Could you check a few things on this model? Use its own coordinates, in mm. Face numbers are marked on the shaded views. A direction names the side the tool comes from. Coordinates: 2 decimals unless noted, no trailing zeros. Loops run counter-clockwise (first coordinate to the right, second up) from the corner with the lowest first, then second, coordinate; pieces in that order, holes last. Notation, with made-up numbers: M -10,30.25 L 30,30.25 A17 ccw 30,50.25 Z; hole C 63.25,4.25 d7. An arc over 180 degrees is marked long. Return JSON: item names as keys, results as strings. Group by question number.
from build123d import *

# Parameters (mm, degrees)
F0_W     = 65
F0_H     = 48.220679
F0_R     = 1.491954
F0_W_2   = 7.12351
F0_H_2   = 5.636183
F0_R_2   = 2.348409
F0_R_3   = 2.019025
F0_W_3   = 6.966946
F0_H_3   = 7.08437
F0_R_4   = 2.712275
F0_W_4   = 5.990132
F0_H_4   = 3.159632
F0_W_5   = 3.225457
F0_H_5   = 6.780042
F0_W_6   = 6.697657
F0_H_6   = 6.365542
F0_W_7   = 6.033428
F0_H_7   = 6.476249
F0_W_8   = 3.155096
F0_H_8   = 2.989037
F0_W_9   = 4.483557
F0_H_9   = 3.376505
F0_W_10  = 5.864762
F0_H_10  = 13.520941
F1_DEPTH = 1.5
F2_DEPTH = 2
F3_DEPTH = 4
F4_DEPTH = 7
F5_W     = 2.606562
F5_H     = 14.894642
F5_W_2   = 2.66153
F5_H_2   = 7.59319
F5_W_3   = 15.029821
F5_H_3   = 2.42669
F5_W_4   = 15.577784
F5_H_4   = 2.504971
F6_DEPTH = 7


with BuildPart() as f1:
    # F0 (on Top) → F1 (new body)
    with BuildSketch(Plane.XY):
        with Locations((15.373986, 7.248863)):
            Rectangle(F0_W, F0_H)
        with Locations((-13.490251, -13.718908)):
            Circle(F0_R, mode=Mode.SUBTRACT)
        with Locations((-6.637482, -5.545355)):
            Rectangle(F0_W_2, F0_H_2, mode=Mode.SUBTRACT)
        with Locations((16.112888, -10.907532)):
            Circle(F0_R_2, mode=Mode.SUBTRACT)
        with Locations((45.080185, -12.724719)):
            Circle(F0_R_3, mode=Mode.SUBTRACT)
        with Locations((33.124202, 5.70149)):
            Rectangle(F0_W_3, F0_H_3, mode=Mode.SUBTRACT)
        with Locations((-12.451392, 11.686808)):
            Circle(F0_R_4, mode=Mode.SUBTRACT)
        with Locations((-5.081796, 11.177822)):
            Rectangle(F0_W_4, F0_H_4, mode=Mode.SUBTRACT)
        with Locations((5.516132, 11.934817)):
            Rectangle(F0_W_5, F0_H_5, mode=Mode.SUBTRACT)
        with Locations((-12.56736, 25.071582)):
            Rectangle(F0_W_6, F0_H_6, mode=Mode.SUBTRACT)
        with Locations((-5.205472, 22.802127)):
            Rectangle(F0_W_7, F0_H_7, mode=Mode.SUBTRACT)
        with Locations((8.798722, 25.099258)):
            Rectangle(F0_W_8, F0_H_8, mode=Mode.SUBTRACT)
        with Locations((1.492187, 25.846517)):
            Rectangle(F0_W_9, F0_H_9, mode=Mode.SUBTRACT)
        with Locations((42.443838, 19.138021)):
            Rectangle(F0_W_10, F0_H_10, mode=Mode.SUBTRACT)
        with Locations((-12.451392, 11.686808)):
            Circle(F0_R_4)
        with Locations((-6.637482, -5.545355)):
            Rectangle(F0_W_2, F0_H_2)
        with Locations((-5.081796, 11.177822)):
            Rectangle(F0_W_4, F0_H_4)
        with Locations((-5.205472, 22.802127)):
            Rectangle(F0_W_7, F0_H_7)
        with Locations((-12.56736, 25.071582)):
            Rectangle(F0_W_6, F0_H_6)
        with Locations((1.492187, 25.846517)):
            Rectangle(F0_W_9, F0_H_9)
        with Locations((5.516132, 11.934817)):
            Rectangle(F0_W_5, F0_H_5)
        with Locations((8.798722, 25.099258)):
            Rectangle(F0_W_8, F0_H_8)
        with Locations((16.112888, -10.907532)):
            Circle(F0_R_2)
        with Locations((33.124202, 5.70149)):
            Rectangle(F0_W_3, F0_H_3)
        with Locations((42.443838, 19.138021)):
            Rectangle(F0_W_10, F0_H_10)
    extrude(amount=-F1_DEPTH)

    # F0 (on Top) → F2 (join)
    with BuildSketch(Plane.XY):
        with Locations((-12.56736, 25.071582)):
            Rectangle(F0_W_6, F0_H_6)
        with Locations((-5.205472, 22.802127)):
            Rectangle(F0_W_7, F0_H_7)
        with Locations((-5.081796, 11.177822)):
            Rectangle(F0_W_4, F0_H_4)
        with Locations((5.516132, 11.934817)):
            Rectangle(F0_W_5, F0_H_5)
        with Locations((1.492187, 25.846517)):
            Rectangle(F0_W_9, F0_H_9)
        with Locations((8.798722, 25.099258)):
            Rectangle(F0_W_8, F0_H_8)
        with Locations((33.124202, 5.70149)):
            Rectangle(F0_W_3, F0_H_3)
        with Locations((-6.637482, -5.545355)):
            Rectangle(F0_W_2, F0_H_2)
    extrude(amount=F2_DEPTH)

    # F0 (on Top) → F3 (join)
    with BuildSketch(Plane.XY):
        with Locations((-12.451392, 11.686808)):
            Circle(F0_R_4)
        with Locations((16.112888, -10.907532)):
            Circle(F0_R_2)
    extrude(amount=F3_DEPTH)

    # F0 (on Top) → F4 (join)
    with BuildSketch(Plane.XY):
        with Locations((42.443838, 19.138021)):
            Rectangle(F0_W_10, F0_H_10)
    extrude(amount=F4_DEPTH)

    # F5 (on face) → F6 (join)
    with BuildSketch(Plane.XY):
        with Locations((11.685232, -5.207297)):
            Rectangle(F5_W, F5_H)
        with Locations((11.835448, 14.843981)):
            Rectangle(F5_W_2, F5_H_2)
        with Locations((20.759405, 28.151636)):
            Rectangle(F5_W_3, F5_H_3)
        with Locations((37.159131, 28.269056)):
            Rectangle(F5_W_4, F5_H_4)
    extrude(amount=F6_DEPTH)


solid = f1.part
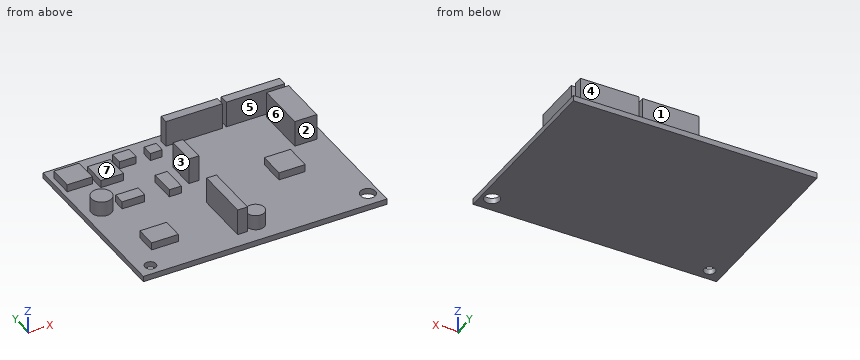
(1) Imagine slicing it at C-C, the plane z = 3.25. Write out the boundary of the cut face in (x, y).
(2) Will these pins go through, and if not, where does the flat tip stop? P1, Ø1.5, axis at x = 1, z = 1.5, coming from the -Y side; P2, Ø2, axis at x = 12, z = 4.5, coming from the +Y side; P3, Ø1.6, axis at y = -6.5, z = 1.5, coming from the +X side.
(3) We'd pull the mould along X, two halves only. Please class the marked faces 6 and 7: +X half, -X half, draft (parallel to the pull), parting line (faces both ways), or undercut.
(4) Imagine slicing it at D-D, the plane x = 21. Write out the boundary of the cut face in (y, z), then the cut area to 3 significant figures.
(5) Imagine slicing it at A-A, the plane x = 32.5. Write out the boundary of the cut face in (y, z).
(6) If I drill on L1, parallel to X at y = 24, z = 0.75; L2, parallel to Y at x = -7, z = 1; L3, parallel to X at y = 17, z = 4, over which ranges is the centre line in solid material (lowest first)? Write a range as [from, to].
(7) For the marked faces 1, 2, 3, 4 and 5, which set-ups out of +Z, -Z, +X, -X, +Y, -Y let a thin tool reach every point of the face, with its end or its side?
(8) Imagine slicing it at B-B, the plane y = -4. Write out the boundary of the cut face in (x, z).
Checks:
{
 "1": {"outline": "C -12.45,11.69 d5.42; M 10.38,-12.65 L 12.99,-12.65 L 12.99,2.24 L 10.38,2.24 Z; M 10.5,11.05 L 13.17,11.05 L 13.17,18.64 L 10.5,18.64 Z; M 13.24,26.94 L 28.27,26.94 L 28.27,29.36 L 13.24,29.36 Z; C 16.11,-10.91 d4.7; M 29.37,27.02 L 44.95,27.02 L 44.95,29.52 L 29.37,29.52 Z; M 39.51,12.38 L 45.38,12.38 L 45.38,25.9 L 39.51,25.9 Z"},
 "2": {"P1": "y = 24.16", "P2": "y = 18.64", "P3": "x = 12.99"},
 "3": {"face 6": "undercut", "face 7": "draft"},
 "4": {"outline": "M -16.86,-1.5 L 31.36,-1.5 L 31.36,0 L 29.36,0 L 29.36,7 L 26.94,7 L 26.94,0 L -16.86,0 Z", "area": "89.3 mm²"},
 "5": {"outline": "M -16.86,-1.5 L 31.36,-1.5 L 31.36,0 L 29.52,0 L 29.52,7 L 27.02,7 L 27.02,0 L 9.24,0 L 9.24,2 L 2.16,2 L 2.16,0 L -16.86,0 Z"},
 "6": {"L1": "[-15.92, -9.22], [-8.22, -2.19], [7.22, 10.38], [39.51, 45.38]", "L2": "[-8.36, -2.73], [9.6, 12.76], [19.56, 26.04]", "L3": "[10.5, 13.17], [39.51, 45.38]"},
 "7": {"face 1": "+Z, -X, +Y", "face 2": "+Z, +X, -Y", "face 3": "+Z, +Y", "face 4": "+Z, +X, -X, +Y", "face 5": "+Z, +X"},
 "8": {"outline": "M -17.13,-1.5 L 47.87,-1.5 L 47.87,0 L 12.99,0 L 12.99,7 L 10.38,7 L 10.38,0 L -3.08,0 L -3.08,2 L -10.2,2 L -10.2,0 L -17.13,0 Z"}
}
